Read the model definition and answer for the solid it produces. Units are mm, in the model's axes. A direction names the side the tool comes from. Coordinates: 2 decimals unless noted, no trailing zeros. Loops run counter-clockwise (first coordinate to the right, second up) from the corner with the lowest first, then second, coordinate; pieces in that order, holes last.
Q1. Flat-ended cylindrical pins translate along their axes: P1, Ø5, axis at x = -33.59, y = 33.59, coming from the +Z side; P2, Ø3, axis at x = 32.5, z = 12, coming from the +Y side; P3, Ø2, axis at x = 32.5, y = -33, coming from the -Z side. Find the tip coordinate at first contact, or state that the pin passes through.
Q2. Straight lines are drawn through the part: line 1 (X direction, y = 222.5, z = 4.4); line 2 (Y direction, x = -23.5, z = 23); line 3 (Y direction, x = -8, z = 2). For each, find the intervals that lie inside material, in ascending order.
Q3. Section A-A (y = 0) is taken. Give the vertices of the cut face in (x, z), then the cut area to 3 significant figures.
Q4. The mould has two halves that part along X. Classify faces 1 (the face through (-33.067, 90.74, 21.036)), 2 (the face through (-40, 103, 29)), 3 (the face through (34.357, 30.122, 1.479)), 4 (the face through (0.87, 237.49, 4.93)): pulls with the +X half, pulls with the -X half, needs draft (parallel to the pull), parting line crosses it, or undercut.
Q5. Section B-B (y = 184.5) is taken. Give the vertices of the cut face in (x, z).
Q6. Which of the six approach directions +Z, -Z, +X, -X, +Y, -Y give full straight-line access (tool end or side, diameter ignored) to faces 5 (the face through (0, 82, 3)), 6 (the face through (6, 195, 5)), 7 (the face through (0, 141.5, 21)), 8 (the face through (-32.602, 144.595, 23.065)), 9 (the face through (32.602, 144.595, 23.065))?
from build123d import *

# Parameters (mm, degrees)
SKETCH1_R               = 20
SKETCH1_R_2             = 7.5
BOSS_EXTRUDE1_DEPTH     = 36.5
SKETCH4_R               = 51.5
CUT_EXTRUDE3_DEPTH      = 31.5
CUT_EXTRUDE4_DEPTH      = 247.841548367
CUT_EXTRUDE4_DEPTH_BACK = 247.841548367
SKETCH5_W               = 26.5
SKETCH5_H               = 90
SHELL1_START            = 6
SHELL1_DEPTH            = 30.5
BOSS_EXTRUDE2_START     = -7.5
SKETCH7_R               = 2
BOSS_EXTRUDE2_DEPTH     = 7.5
BOSS_EXTRUDE3_DEPTH     = 15
CUT_EXTRUDE5_DEPTH      = 247.025913269
CUT_EXTRUDE5_DEPTH_BACK = 6
SKETCH9_R               = 1.6
SKETCH9_W               = 30
SKETCH9_H               = 15
FILLET1_R               = 10
FILLET2_R               = 5
SKETCH10_R              = 1.55
CUT_EXTRUDE6_DEPTH      = 10
SKETCH11_OUTSIDE_W      = 178.416
SKETCH11_OUTSIDE_H      = 359.416
SKETCH11_OUTSIDE_R      = 3.55
CUT_EXTRUDE8_DEPTH      = 3
SKETCH12_R              = 12.1
CUT_EXTRUDE9_DEPTH      = 5
SKETCH13_R              = 2.25
CUT_EXTRUDE10_DEPTH     = 6


# Read off the part's stored shape, not the designer's step: Shell1
with BuildPart() as part:
    # Sketch1 → Boss-Extrude1 (new body)
    with BuildSketch(Plane.XY):
        with BuildLine():
            ThreePointArc((-54.352625843, 15.42861186), (0, -56.5), (54.352625843, 15.42861186))
            ThreePointArc((54.352625843, 15.42861186), (37.535595393, 105.258460348), (37.34995219, 196.64872093))
            ThreePointArc((37.34995219, 196.64872093), (0, 237.5), (-37.34995219, 196.64872093))
            ThreePointArc((-37.34995219, 196.64872093), (-37.535595393, 105.258460348), (-54.352625843, 15.42861186))
        make_face()
        Circle(SKETCH1_R, mode=Mode.SUBTRACT)
        with Locations((0, 200)):
            Circle(SKETCH1_R_2, mode=Mode.SUBTRACT)
    extrude(amount=BOSS_EXTRUDE1_DEPTH)

    # Sketch4 → Cut-Extrude3 (cut)
    with BuildSketch(Plane.XY.offset(36.5)):
        Circle(SKETCH4_R)
    extrude(amount=-CUT_EXTRUDE3_DEPTH, mode=Mode.SUBTRACT)

    # Sketch5 → Cut-Extrude4 (cut, two sides: drawn at the far end of the back side and taken through both)
    with BuildSketch(Plane(origin=(0, 0, 0), x_dir=(0, 0, -1), z_dir=(1, 0, 0)).offset(-CUT_EXTRUDE4_DEPTH_BACK)):
        with Locations((-23.25, 192.5)):
            Rectangle(SKETCH5_W, SKETCH5_H)
    extrude(amount=CUT_EXTRUDE4_DEPTH + CUT_EXTRUDE4_DEPTH_BACK, mode=Mode.SUBTRACT)

    # Shell1 outline → Shell1 (cut)
    with BuildSketch(Plane.XY.offset(SHELL1_START)):
        with BuildLine():
            ThreePointArc((-42.077009937, 39.188968279), (0, 57.5), (42.077009937, 39.188968279))
            ThreePointArc((42.077009937, 39.188968279), (33.155030313, 90.022278833), (29.457543912, 141.5))
            Line((29.457543912, 141.5), (-29.457543912, 141.5))
            ThreePointArc((-29.457543912, 141.5), (-33.155030313, 90.022278833), (-42.077009937, 39.188968279))
        make_face()
    extrude(amount=SHELL1_DEPTH, mode=Mode.SUBTRACT)

    # Sketch7 → Boss-Extrude2 (add)
    # profile 1 of 2: a face of its own
    with BuildSketch(Plane.XY.offset(36.5).offset(BOSS_EXTRUDE2_START)):
        with BuildLine():
            Line((-39.159181835, 90.358571571), (-46.159181835, 97.5))
            Line((-46.159181835, 97.5), (-46.159181835, 112.5))
            Line((-46.159181835, 112.5), (-36.669554937, 115.653883533))
            ThreePointArc((-36.669554937, 115.653883533), (-37.753606302, 102.990404952), (-39.159181835, 90.358571571))
        make_face()
        with Locations((-42.159181835, 105)):
            Circle(SKETCH7_R, mode=Mode.SUBTRACT)
    # profile 2 of 2: a face of its own
    with BuildSketch(Plane.XY.offset(36.5).offset(BOSS_EXTRUDE2_START)):
        with BuildLine():
            Line((46.159181835, 97.5), (46.159181835, 112.5))
            Line((46.159181835, 112.5), (36.669554937, 115.653883533))
            ThreePointArc((36.669554937, 115.653883533), (37.753606302, 102.990404952), (39.159181835, 90.358571571))
            Line((39.159181835, 90.358571571), (46.159181835, 97.5))
        make_face()
        with Locations(Location((42.159181835, 105, 0), (0, 0, 180))):
            Circle(SKETCH7_R, mode=Mode.SUBTRACT)
    extrude(amount=BOSS_EXTRUDE2_DEPTH)

    # Sketch8 → Boss-Extrude3 (add)
    with BuildSketch(Plane.XY.offset(6)):
        with BuildLine():
            Line((-35.707844492, 72), (-25.707844492, 72))
            Line((-25.707844492, 72), (-25.707844492, 69.5))
            Line((-25.707844492, 69.5), (-36.114376268, 69.5))
            ThreePointArc((-36.114376268, 69.5), (-35.909546125, 70.749745632), (-35.707844492, 72))
        make_face()
        with BuildLine():
            Line((-36.705134195, 66), (-25.707844492, 66))
            Line((-25.707844492, 66), (-25.707844492, 63))
            Line((-25.707844492, 63), (-37.231629056, 63))
            ThreePointArc((-37.231629056, 63), (-36.966124321, 64.499603847), (-36.705134195, 66))
        make_face()
        with BuildLine():
            Line((25.707844492, 63), (37.231629056, 63))
            ThreePointArc((37.231629056, 63), (36.966124321, 64.499603847), (36.705134195, 66))
            Line((36.705134195, 66), (25.707844492, 66))
            Line((25.707844492, 66), (25.707844492, 63))
        make_face()
        with BuildLine():
            Line((25.707844492, 69.5), (36.114376268, 69.5))
            ThreePointArc((36.114376268, 69.5), (35.909546125, 70.749745632), (35.707844492, 72))
            Line((35.707844492, 72), (25.707844492, 72))
            Line((25.707844492, 72), (25.707844492, 69.5))
        make_face()
    extrude(amount=BOSS_EXTRUDE3_DEPTH)

    # Sketch9 → Cut-Extrude5 (cut, two sides: drawn at the far end of the back side and taken through both)
    with BuildSketch(Plane.XY.offset(6).offset(-CUT_EXTRUDE5_DEPTH_BACK)):
        with Locations((-7, 77)):
            Circle(SKETCH9_R)
        with Locations((7, 77)):
            Circle(SKETCH9_R)
        with Locations((0, 89.5)):
            Rectangle(SKETCH9_W, SKETCH9_H)
    extrude(amount=CUT_EXTRUDE5_DEPTH + CUT_EXTRUDE5_DEPTH_BACK, mode=Mode.SUBTRACT)

    # Fillet1
    fillet1_edges = [part.edges().sort_by_distance(p)[0] for p in [
        (35.369251346, 147.5, 23.25),
        (-35.369251346, 147.5, 23.25),
    ]]
    fillet(fillet1_edges, radius=FILLET1_R)

    # Fillet2
    fillet2_edges = [part.edges().sort_by_distance(p)[0] for p in [
        (15, 97, 3),
        (15, 82, 3),
        (-15, 82, 3),
        (-15, 97, 3),
    ]]
    fillet(fillet2_edges, radius=FILLET2_R)

    # Sketch10 → Cut-Extrude6 (cut)
    with BuildSketch(Plane.XY.offset(5)):
        with Locations((-33.587572106, 33.587572106)):
            Circle(SKETCH10_R)
        with Locations((33.587572106, 33.587572106)):
            Circle(SKETCH10_R)
        with Locations((33.587572106, -33.587572106)):
            Circle(SKETCH10_R)
        with Locations((-33.587572106, -33.587572106)):
            Circle(SKETCH10_R)
    extrude(amount=-CUT_EXTRUDE6_DEPTH, mode=Mode.SUBTRACT)

    # Sketch11 outside → Cut-Extrude8 (cut)
    # profile 1 of 5: a face of its own
    with BuildSketch(Plane(origin=(0, 0, 0), x_dir=(-1, 0, 0), z_dir=(0, 0, -1))):
        with Locations((0, 90.5)):
            Rectangle(SKETCH11_OUTSIDE_W, SKETCH11_OUTSIDE_H)
        with BuildLine():
            ThreePointArc((37.34995219, 196.64872093), (37.535595393, 105.258460348), (54.352625843, 15.42861186))
            ThreePointArc((54.352625843, 15.42861186), (0, -56.5), (-54.352625843, 15.42861186))
            ThreePointArc((-54.352625843, 15.42861186), (-37.535595393, 105.258460348), (-37.34995219, 196.64872093))
            ThreePointArc((-37.34995219, 196.64872093), (0, 237.5), (37.34995219, 196.64872093))
        make_face(mode=Mode.SUBTRACT)
    # profile 2 of 5: a face of its own
    with BuildSketch(Plane(origin=(0, 0, 0), x_dir=(-1, 0, 0), z_dir=(0, 0, -1))):
        with Locations((-33.587572106, -33.587572106)):
            Circle(SKETCH11_OUTSIDE_R)
    # profile 3 of 5: a face of its own
    with BuildSketch(Plane(origin=(0, 0, 0), x_dir=(-1, 0, 0), z_dir=(0, 0, -1))):
        with Locations((33.587572106, -33.587572106)):
            Circle(SKETCH11_OUTSIDE_R)
    # profile 4 of 5: a face of its own
    with BuildSketch(Plane(origin=(0, 0, 0), x_dir=(-1, 0, 0), z_dir=(0, 0, -1))):
        with Locations((33.587572106, 33.587572106)):
            Circle(SKETCH11_OUTSIDE_R)
    # profile 5 of 5: a face of its own
    with BuildSketch(Plane(origin=(0, 0, 0), x_dir=(-1, 0, 0), z_dir=(0, 0, -1))):
        with Locations((-33.587572106, 33.587572106)):
            Circle(SKETCH11_OUTSIDE_R)
    extrude(amount=-CUT_EXTRUDE8_DEPTH, mode=Mode.SUBTRACT)

    # Sketch12 → Cut-Extrude9 (cut)
    with BuildSketch(Plane(origin=(0, 0, 0), x_dir=(-1, 0, 0), z_dir=(0, 0, -1))):
        with Locations((0, 200)):
            Circle(SKETCH12_R)
    extrude(amount=-CUT_EXTRUDE9_DEPTH, mode=Mode.SUBTRACT)

    # Sketch13 → Cut-Extrude10 (cut)
    with BuildSketch(Plane(origin=(0, 0, 0), x_dir=(-1, 0, 0), z_dir=(0, 0, -1))):
        with Locations((0, 222.5)):
            Circle(SKETCH13_R)
        with Locations((22.5, 200)):
            Circle(SKETCH13_R)
        with Locations((0, 177.5)):
            Circle(SKETCH13_R)
        with Locations((-22.5, 200)):
            Circle(SKETCH13_R)
    extrude(amount=-CUT_EXTRUDE10_DEPTH, mode=Mode.SUBTRACT)


solid = part.part
Numbers:
1. P1: stops at z = 5
1. P2: stops at y = 145.89
1. P3: stops at z = 3
2. line 1: x = -30 to -2.25, 2.25 to 30
2. line 2: y = -51.38 to -45.83, 45.83 to 52.48, 141.5 to 147.5
2. line 3: y = -55.93 to -18.33, 18.33 to 75.75, 78.25 to 82, 97 to 190.92, 209.08 to 236.64
3. outline: (-56.5, 0) - (-20, 0) - (-20, 5) - (-51.5, 5) - (-51.5, 36.5) - (-56.5, 36.5) - close; (20, 0) - (56.5, 0) - (56.5, 36.5) - (51.5, 36.5) - (51.5, 5) - (20, 5) - close
3. area: 680 mm2
4. face 1: undercut
4. face 2: needs draft
4. face 3: undercut
4. face 4: parting line crosses it
5. outline: (-36.41, 0) - (36.41, 0) - (36.41, 10) - (-36.41, 10) - close
6. face 5: +Z, -Z
6. face 6: -Z
6. face 7: +Z
6. face 8: +Z, -X, +Y
6. face 9: +Z, +X, +Y
